Here's how the part is built. I have some questions about the finished solid (model axes, mm). Face numbers are marked on the shaded views. A direction names the side the tool comes from. Round coordinates to 2 decimals unless told otherwise and drop trailing zeros. Loops run counter-clockwise (first coordinate to the right, second up) from the corner with the lowest first, then second, coordinate; pieces in that order, holes last. Notation, with made-up numbers: M 40,56.25 L 71,56.25 A15 cw 71,69.25 Z; hole C 28,-40 d9. An arc over 180 degrees is marked long. Write each question's results on one line, items separated by ' | '. Start each with the question number.
```python
from build123d import *

# Parameters (mm, degrees)
F1_DEPTH    = 50
F3_R        = 2
F4_R        = 3
F5_R        = 2
F6_R        = 3
F7_T1_DEPTH = 54.0990195136
F7_T3_DEPTH = 56.0990195136
F8_R        = 10


# Not quite as in the source:
# - a fillet or chamfer that OpenCascade refuses, or shapes differently, is made with other operations: its cross-section is extruded or revolved along the edge and cut away or added


with BuildPart() as f1:
    # F0 (on Top) → F1 (new body)
    with BuildSketch(Plane.XY):
        Polygon((6, 0), (0, 0), (0, -2), (8.1142857143, -2), (6, 35), (7, 40), (5, 40), (4, 35), align=None)
    extrude(amount=F1_DEPTH)

    # F2: F1 across face


with BuildPart() as f1_1:
    add(f1.part)
    add(f1.part.mirror(Plane(origin=(0, -1, 25), x_dir=(0, -1, 0), z_dir=(-1, 0, 0))))

    # F3
    f3_edges = [f1_1.edges().sort_by_distance(p)[0] for p in [
        (6, 0, 25),
    ]]
    fillet(f3_edges, radius=F3_R)

    # F4
    f4_edges = [f1_1.edges().sort_by_distance(p)[0] for p in [
        (8.114286, -2, 25),
    ]]
    fillet(f4_edges, radius=F4_R)

    # F5
    f5_edges = [f1_1.edges().sort_by_distance(p)[0] for p in [
        (-6, 0, 25),
    ]]
    fillet(f5_edges, radius=F5_R)

    # F6
    f6_edges = [f1_1.edges().sort_by_distance(p)[0] for p in [
        (-8.114286, -2, 25),
    ]]
    fillet(f6_edges, radius=F6_R)

    # F7: fillet of radius 1 on 4 edges, made by hand

    # F7_s2 → F7_t1 (cut)
    with BuildSketch(Plane.XY.offset(-2.0495097568)):
        with BuildLine():
            ThreePointArc((-5.8198039027, 40), (-5.1858149971, 39.7733421413), (-4.839223227, 39.1961161351))
            Line((-4.839223227, 39.1961161351), (-5, 40))
            Line((-5, 40), (-5.8198039027, 40))
        make_face()
        with BuildLine():
            ThreePointArc((5.8198039027, 40), (5.1858149971, 39.7733421413), (4.839223227, 39.1961161351))
            Line((4.839223227, 39.1961161351), (5, 40))
            Line((5, 40), (5.8198039027, 40))
        make_face()
    extrude(amount=F7_T1_DEPTH, mode=Mode.SUBTRACT)

    # F7_s4 → F7_t3 (cut)
    with BuildSketch(Plane.XY.offset(-3.0495097568)):
        with BuildLine():
            ThreePointArc((-6.760776773, 38.8038838649), (-6.5535382386, 39.6339889056), (-5.7801960973, 40))
            Line((-5.7801960973, 40), (-7, 40))
            Line((-7, 40), (-6.760776773, 38.8038838649))
        make_face()
        with BuildLine():
            ThreePointArc((6.760776773, 38.8038838649), (6.5535382386, 39.6339889056), (5.7801960973, 40))
            Line((5.7801960973, 40), (7, 40))
            Line((7, 40), (6.760776773, 38.8038838649))
        make_face()
    extrude(amount=F7_T3_DEPTH, mode=Mode.SUBTRACT)

    # F8
    f8_edges = [f1_1.edges().sort_by_distance(p)[0] for p in [
        (-4, 35, 25),
        (4, 35, 25),
        (6, 35, 25),
        (-6, 35, 25),
    ]]
    fillet(f8_edges, radius=F8_R)


solid = f1_1.part
```
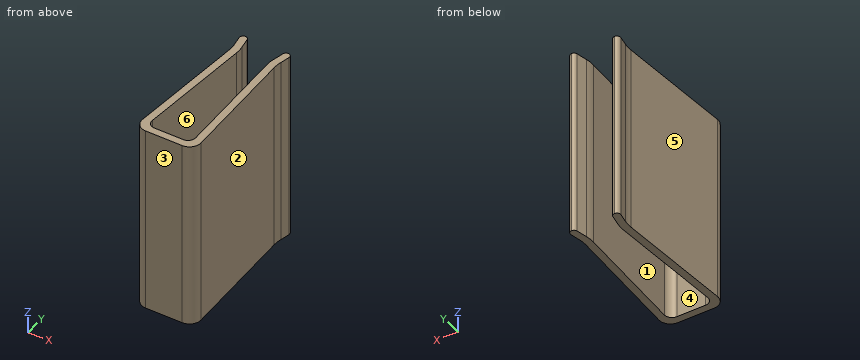
Item 1: I need wall thicknesses on L1, parallel to X at y = 34.5, z = 12.5; L2, parallel to X at y = 18, z = 48; L3, parallel to Y at x = -0.5, z = 7. Which ranges of each line are inside material? Lowest first, please.
Item 2: If we section it at B-B on y = 28.5: Please give me the cut outline in (x, z), and give its area (3 significant figures).
Item 3: If we section it at C-C on x = 0.75: Please give me the cut outline in (y, z), and give its area (3 significant figures).
Item 4: Which directions (+Z, -Z, +X, -X, +Y, -Y) give clear straight access to the entire face, cutting with the end or side of a thin tool? Please do the marked faces 1 and 2.
Item 5: If we mould it in two halves opening along Y, with no side actions, what happens to the marked faces 3, 4, 5 and 6? For each: released by +Y, released by -Y, zero draft, split by the parting line, or undercut.
Item 6: I'm going to push flat-ended pins straight in: pin 1 (10 mm diameter, centred on y = 6.5, z = 17.5, fed in from -X); pin 2 (4 mm diameter, centred on x = -2, z = 17, fed in from +Y). Where does each tip first touch, or does it pass through?
Item 7: If we section it at A-A on z = 6: Please give me the cut outline in (x, y), and give its area (3 significant figures).
Numbers:
1) L1: -6.06 to -4.06, 4.06 to 6.06 | L2: -6.97 to -4.97, 4.97 to 6.97 | L3: -2 to 0
2) outline: M -6.37,0 L -4.37,0 L -4.37,50 L -6.37,50 Z; M 4.37,0 L 6.37,0 L 6.37,50 L 4.37,50 Z | area: 200 mm²
3) outline: M -2,0 L 0,0 L 0,50 L -2,50 Z | area: 100 mm²
4) face 1: +Z, -Z | face 2: +Z, -Z, +X
5) face 3: released by -Y | face 4: released by +Y | face 5: undercut | face 6: undercut
6) pin 1: x = -7.91 | pin 2: y = 0
7) outline: M -7.93,1.17 A3 ccw -4.94,-2 L 4.94,-2 A3 ccw 7.93,1.17 L 6.07,33.72 A10 cw 6.25,36.25 L 6.76,38.8 A1 ccw 5.8,40 A1 ccw 4.84,39.2 L 4.25,36.25 A10 ccw 4.07,33.72 L 5.88,2.11 A2 cw 3.88,0 L -3.88,0 A2 cw -5.88,2.11 L -4.07,33.72 A10 ccw -4.25,36.25 L -4.84,39.2 A1 ccw -5.8,40 A1 ccw -6.76,38.8 L -6.25,36.25 A10 cw -6.07,33.72 Z | area: 189 mm²
